Can you work these out from the model? Positions are in its coordinate system, mm. Face numbers are marked on the shaded views. Coordinates: 2 decimals unless noted, no trailing zeros. Order: outer loops, then holes, each group sorted by start corner. A loop starts at its lowest first (then second) coordinate and runs counter-clockwise, first axis right, second up.
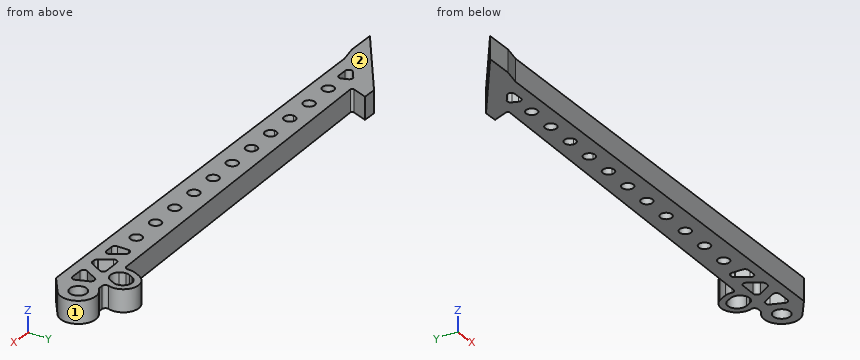
```python
from build123d import *

# Parameters (mm, degrees)
SKETCH1_R           = 3.2639
SKETCH1_R_2         = 4.8025
BOSS_EXTRUDE1_DEPTH = 12.7
EXTRUDE_THIN1_DEPTH = 12.7
FILLET6_R           = 2
FILLET3_R           = 1
FILLET4_R           = 2
BOSS_EXTRUDE5_DEPTH = 12.7
CUT_EXTRUDE8_DEPTH  = 12.7
FILLET13_R          = 100
FILLET14_R          = 2
CUT_EXTRUDE9_DEPTH  = 12.7
FILLET16_R          = 2
BOSS_EXTRUDE6_DEPTH = 12.7
SKETCH18_R          = 3.2639
CUT_EXTRUDE10_DEPTH = 12.7
FILLET17_R          = 2


with BuildPart() as part:
    # Sketch1 → Boss-Extrude1 (new body)
    with BuildSketch(Plane.XY):
        with BuildLine():
            Line((-266.801436578, 66.762186411), (-251.101436578, 66.762186411))
            Line((-251.101436578, 66.762186411), (-241.101436578, 68.762186411))
            Line((-241.101436578, 68.762186411), (18.198563422, 71.262186411))
            Line((18.198563422, 71.262186411), (29.067448443, 79.140508783))
            ThreePointArc((29.067448443, 79.140508783), (30.773671377, 93.765412775), (16.057134994, 94.237186411))
            Line((16.057134994, 94.237186411), (-218.528848369, 87.762186411))
            Line((-218.528848369, 87.762186411), (-214.528848369, 97.762186411))
            Line((-214.528848369, 97.762186411), (-222.528848369, 97.762186411))
            Line((-222.528848369, 97.762186411), (-266.801436578, 66.762186411))
        make_face()
        with Locations((-211.801436578, 78.496276476)):
            Circle(SKETCH1_R, mode=Mode.SUBTRACT)
        with BuildLine():
            ThreePointArc((-197.554771535, 78.761405302), (-194.352166872, 82.085470554), (-191.028101621, 78.882865891))
            ThreePointArc((-191.028101621, 78.882865891), (-194.230706283, 75.55880064), (-197.554771535, 78.761405302))
        make_face(mode=Mode.SUBTRACT)
        with BuildLine():
            ThreePointArc((-180.044771535, 79.087264423), (-176.842166872, 82.411329675), (-173.518101621, 79.208725013))
            ThreePointArc((-173.518101621, 79.208725013), (-176.720706283, 75.884659761), (-180.044771535, 79.087264423))
        make_face(mode=Mode.SUBTRACT)
        with BuildLine():
            ThreePointArc((-162.534771535, 79.413123544), (-159.332166872, 82.737188796), (-156.008101621, 79.534584134))
            ThreePointArc((-156.008101621, 79.534584134), (-159.210706283, 76.210518882), (-162.534771535, 79.413123544))
        make_face(mode=Mode.SUBTRACT)
        with BuildLine():
            ThreePointArc((-145.024771535, 79.738982665), (-141.822166872, 83.063047917), (-138.498101621, 79.860443255))
            ThreePointArc((-138.498101621, 79.860443255), (-141.700706283, 76.536378003), (-145.024771535, 79.738982665))
        make_face(mode=Mode.SUBTRACT)
        with Locations((-124.251436578, 80.125572081)):
            Circle(SKETCH1_R, mode=Mode.SUBTRACT)
        with Locations((-106.744467891, 80.45137479)):
            Circle(SKETCH1_R, mode=Mode.SUBTRACT)
        with Locations((-89.237499204, 80.777177499)):
            Circle(SKETCH1_R, mode=Mode.SUBTRACT)
        with Locations((-71.727499204, 81.10303662)):
            Circle(SKETCH1_R, mode=Mode.SUBTRACT)
        with BuildLine():
            ThreePointArc((-56.754762895, 76.539814612), (-61.641816892, 81.290680691), (-56.935012167, 86.220185184))
            Line((-56.935012167, 86.220185184), (11.656299, 88.113430183))
            Line((11.656299, 88.113430183), (15.733532107, 77.238699061))
            Line((15.733532107, 77.238699061), (-56.754762895, 76.539814612))
        make_face(mode=Mode.SUBTRACT)
        with Locations((23.198563422, 87.237186411)):
            Circle(SKETCH1_R_2, mode=Mode.SUBTRACT)
    extrude(amount=BOSS_EXTRUDE1_DEPTH)

    # Sketch3 → Extrude-Thin1 (add)
    with BuildSketch(Plane.XY.offset(12.7)):
        Polygon((4.238515695, 91.06458037), (3.224088624, 89.340939538), (-3.171442721, 78.474116994), (-4.185869793, 76.750476162), (0.554142495, 73.960801716), (1.568569566, 75.684442548), (7.964100911, 86.551265092), (8.978527982, 88.274905924), align=None)
        Polygon((-7.406763076, 76.778305642), (-8.483669151, 78.463616684), (-15.08355213, 88.792145717), (-16.160458205, 90.477456759), (-20.795063569, 87.515965054), (-19.718157494, 85.830654012), (-13.118274515, 75.502124979), (-12.04136844, 73.816813937), align=None)
        Polygon((-55.789995158, 86.920345113), (-54.713089083, 85.235034072), (-48.113206103, 74.906505038), (-47.036300029, 73.221193997), (-42.401694665, 76.182685702), (-43.478600739, 77.867996743), (-50.078483719, 88.196525777), (-51.155389794, 89.881836818), align=None)
        Polygon((-30.756415894, 90.46896043), (-31.770842965, 88.745319598), (-38.16637431, 77.878497054), (-39.180801381, 76.154856222), (-34.440789094, 73.365181776), (-33.426362022, 75.088822608), (-27.030830678, 85.955645152), (-26.016403606, 87.679285984), align=None)
    extrude(amount=-EXTRUDE_THIN1_DEPTH)

    # Fillet6
    fillet6_edges = [part.edges().sort_by_distance(p)[0] for p in [
        (-7.55746183, 77.014142621, 6.35),
        (-14.193924314, 87.399916982, 6.35),
        (-38.852657232, 76.712414937, 6.35),
        (-32.865984778, 86.884534137, 6.35),
        (-32.434398171, 76.774295568, 6.35),
        (-26.378761772, 87.063593296, 6.35),
        (-49.203405679, 76.61261983, 6.35),
        (-55.370195509, 86.263376972, 6.35),
        (-42.716385675, 76.675163409, 6.35),
        (-48.956334512, 86.440411206, 6.35),
        (15.733532107, 77.238699061, 6.35),
        (11.656299, 88.113430183, 6.35),
        (-4.010566108, 77.048339456, 6.35),
        (2.350483264, 87.856572736, 6.35),
        (2.407692953, 77.110220087, 6.35),
        (8.83770627, 88.035631895, 6.35),
    ]]
    fillet(fillet6_edges, radius=FILLET6_R)

    # Fillet3
    fillet3_edges = [part.edges().sort_by_distance(p)[0] for p in [
        (-218.528848369, 87.762186411, 6.35),
    ]]
    fillet(fillet3_edges, radius=FILLET3_R)

    # Fillet4
    fillet4_edges = [part.edges().sort_by_distance(p)[0] for p in [
        (-222.528848369, 97.762186411, 6.35),
    ]]
    fillet(fillet4_edges, radius=FILLET4_R)

    # Sketch15 → Boss-Extrude5 (add)
    with BuildSketch(Plane(origin=(0, 0, 0), x_dir=(-1, 0, 0), z_dir=(0, 0, -1))):
        with BuildLine():
            ThreePointArc((-10.240564525, 95.177858348), (-9.91771052, 94.625214052), (-9.618412164, 94.059465945))
            Line((-9.618412164, 94.059465945), (-5.586658581, 93.948182209))
            ThreePointArc((-5.586658581, 93.948182209), (-6.060393003, 94.847345318), (-6.352002714, 95.820937828))
            ThreePointArc((-6.352002714, 95.820937828), (-4.888389862, 104.071201116), (2.646503395, 100.405905698))
            ThreePointArc((2.646503395, 100.405905698), (3.686135654, 98.752465403), (4.04944042, 96.833426662))
            ThreePointArc((4.04944042, 96.833426662), (3.785365476, 95.18933076), (3.019706577, 93.710630871))
            Line((3.019706577, 93.710630871), (7.309930071, 93.592212896))
            ThreePointArc((7.309930071, 93.592212896), (7.772330748, 96.70964865), (7.106994943, 99.790159701))
            ThreePointArc((7.106994943, 99.790159701), (6.028678087, 102.129209778), (4.770165569, 104.37644558))
            ThreePointArc((4.770165569, 104.37644558), (-7.334493094, 107.282517011), (-10.240564525, 95.177858348))
        make_face()
    extrude(amount=-BOSS_EXTRUDE5_DEPTH)

    # Sketch15<3> → Cut-Extrude8 (cut)
    with BuildSketch(Plane(origin=(0, 0, 0), x_dir=(-1, 0, 0), z_dir=(0, 0, -1))):
        with BuildLine():
            Line((3.019706577, 93.710630871), (-5.586658581, 93.948182209))
            ThreePointArc((-5.586658581, 93.948182209), (-1.345413965, 91.585425404), (3.019706577, 93.710630871))
        make_face()
    extrude(amount=-CUT_EXTRUDE8_DEPTH, mode=Mode.SUBTRACT)

    # Fillet13
    fillet13_edges = [part.edges().sort_by_distance(p)[0] for p in [
        (6.352002714, 95.820937828, 6.35),
        (-2.646503395, 100.405905698, 6.35),
    ]]
    fillet(fillet13_edges, radius=FILLET13_R)

    # Fillet14
    fillet14_edges = [part.edges().sort_by_distance(p)[0] for p in [
        (16.057134994, 94.237186411, 6.35),
        (-7.309930071, 93.592212896, 6.35),
        (9.618412164, 94.059465945, 6.35),
    ]]
    fillet(fillet14_edges, radius=FILLET14_R)

    # Sketch17 → Cut-Extrude9 (cut)
    with BuildSketch(Plane(origin=(0, 0, 0), x_dir=(-1, 0, 0), z_dir=(0, 0, -1))):
        Polygon((225.771163147, 83.894534568), (237.695045428, 75.54534231), (222.695045428, 75.689962442), align=None)
    extrude(amount=-CUT_EXTRUDE9_DEPTH, mode=Mode.SUBTRACT)

    # Fillet16
    fillet16_edges = [part.edges().sort_by_distance(p)[0] for p in [
        (-237.695045428, 75.54534231, 6.35),
        (-225.771163147, 83.894534568, 6.35),
        (-222.695045428, 75.689962442, 6.35),
    ]]
    fillet(fillet16_edges, radius=FILLET16_R)

    # Sketch20 → Boss-Extrude6 (add)
    with BuildSketch(Plane(origin=(0, 0, 0), x_dir=(-1, 0, 0), z_dir=(0, 0, -1))):
        Polygon((24.344481835, 87.119743124), (24.344481835, 76.852293218), (33.994868443, 72.80053303), (65.802348689, 76.852293218), (61.329456715, 89.562181047), align=None)
    extrude(amount=-BOSS_EXTRUDE6_DEPTH)

    # Sketch18 → Cut-Extrude10 (cut)
    with BuildSketch(Plane(origin=(0, 0, 0), x_dir=(-1, 0, 0), z_dir=(0, 0, -1))):
        with Locations((54.220530518, 81.428839328)):
            Circle(SKETCH18_R)
        with Locations((36.713561831, 81.754642037)):
            Circle(SKETCH18_R)
    extrude(amount=-CUT_EXTRUDE10_DEPTH, mode=Mode.SUBTRACT)

    # Fillet17
    fillet17_edges = [part.edges().sort_by_distance(p)[0] for p in [
        (-14.044481835, 76.951599042, 6.35),
        (-20.607785311, 87.222882748, 6.35),
        (-24.344481835, 76.852293218, 6.35),
        (-24.344481835, 87.119743124, 6.35),
    ]]
    fillet(fillet17_edges, radius=FILLET17_R)


solid = part.part
```
1. I'm going to push flat-ended pins straight in: pin 1 (2 mm diameter, centred on y = 98.5, z = 7.5, fed in from +X); pin 2 (5 mm diameter, centred on y = 82, z = 4.5, fed in from +X); pin 3 (6 mm diameter, centred on x = -162.5, z = 4.5, fed in from -Y). Where does each tip first touch, or does it pass through?
Completed:
pin 1: stops at x = 11.53
pin 2: stops at x = 32.82
pin 3: stops at y = 69.49
2. Thinking about a two-plate mould opening in X: for the marked faces 1 and 2, which applies, pulls with the +X half, pulls with the -X half, needs draft (parallel to the pull), parting line crosses it, or undercut?
Completed:
face 1: undercut
face 2: needs draft
3. Imagine slicing it at A-A on x = -205.5. Please give me the cut outline in (y, z).
Completed:
outline: (69.11, 0) - (88.12, 0) - (88.12, 12.7) - (69.11, 12.7) - close
4. Please list where these lines run through material, in increasing order: probe 1 along X at (y, z) = (95.5, 1); probe 2 along X at (y, z) = (86.5, 11.5); probe 3 along X at (y, z) = (86, 10).
Completed:
probe 1: x = -225.76 to -215.43, -7.74 to -3.88, 6.4 to 11.02, 17.57 to 28.83
probe 2: x = -238.61 to -23.84, -20.17 to -12.34, 0.65 to 7.93, 12.26 to 18.45, 27.94 to 33.17
probe 3: x = -239.33 to -24.17, -19.83 to -12.54, 0.78 to 7.64, 12.45 to 18.56, 27.84 to 33.12
5. Imagine slicing it at B-B on z = 6.75. Give the number of separate pieces and of enclosed holes in the cut face, then the cut area to 3 significant figures.
Completed:
separate pieces: 1
enclosed holes: 17
area: 5,380 mm2
6. Imagine slicing it at C-C on x = -169.5. Please give me the cut outline in (y, z).
Completed:
outline: (69.45, 0) - (89.12, 0) - (89.12, 12.7) - (69.45, 12.7) - close
